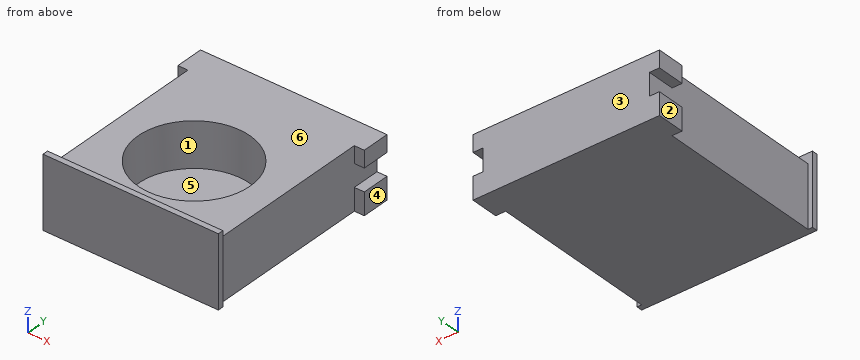
from build123d import *

# Parameters (mm, degrees)
F0_W     = 18.923
F0_H     = 6.985
F1_DEPTH = 22.86
F3_DEPTH = 0.635
F4_R     = 6.35
F5_DEPTH = 5.08
F4_W     = 1.143
F4_H     = 3.175
F6_DEPTH = 6.985
F7_W     = 1.143
F7_H     = 2.54
F8_DEPTH = 12.7


with BuildPart() as f1:
    # F0 (on Front) → F1 (new body)
    with BuildSketch(Plane.XZ):
        with Locations((0, -0.3175)):
            Rectangle(F0_W, F0_H)
    extrude(amount=F1_DEPTH)

    # F2 (on face) → F3 (join)
    with BuildSketch(Plane.XZ.offset(22.86)):
        Polygon((9.976428, 4.318), (-9.9695, 4.318), (-9.9695, -3.81), (-9.4615, -3.81), (-9.4615, 3.175), (9.4615, 3.175), (9.4615, -3.81), (9.976428, -3.81), align=None)
    extrude(amount=-F3_DEPTH)

    # F4 (on face) → F5 (cut)
    with BuildSketch(Plane.XY.offset(3.175)):
        with Locations((0, -13.97)):
            Circle(F4_R)
    extrude(amount=-F5_DEPTH, mode=Mode.SUBTRACT)

    # F4 (on face) → F6 (join, through all)
    with BuildSketch(Plane.XY.offset(3.175)):
        with Locations((-10.033, -1.5875)):
            Rectangle(F4_W, F4_H)
        with Locations((10.033, -1.5875)):
            Rectangle(F4_W, F4_H)
    extrude(amount=-F6_DEPTH)

    # F7 (on face) → F8 (cut)
    with BuildSketch(Plane.XZ):
        with Locations((10.033, 0)):
            Rectangle(F7_W, F7_H)
        with Locations((-10.033, 0)):
            Rectangle(F7_W, F7_H)
    extrude(amount=F8_DEPTH, mode=Mode.SUBTRACT)


solid = f1.part
Verification items for the finished model (mm, model axes). Face numbers are marked on the shaded views. A direction names the side the tool comes from. Give positions to 0.01 mm unless a question says otherwise; leave off trailing zeros. Order: outer loops, then holes, each group sorted by start corner. A loop starts at its lowest first (then second) coordinate and runs counter-clockwise, first axis right, second up. Notation, with made-up numbers: M -39,-3.75 L 11,-3.75 A11 ccw 11,14.25 Z; hole C -12.5,79.25 d8. An arc over 180 degrees is marked long. Answer as a JSON object with one key per item and string values. Group by question number.
1) Cross-section at D-D (x = -8.75). Enter the section's corners in (y, z) (3 decimals).
2) Depth check by flat-ended pin: pin 1 Ø1.3 at (x, z) = (10, -3) entering from -Y; pin 2 Ø4 at (y, z) = (-17.5, -2.5) entering from +X; pin 3 Ø0.6 at (x, y) = (10, -2) entering from +Z (3 decimals); pin 4 Ø1.5 at (y, z) = (-8.5, -3) entering from -X. Enter the tip coordinate at first touch or a pass-through.
3) Cross-section at A-A (x = 0). Enter the section's corners in (y, z) (3 decimals), then the cut area to 3 significant figures.
4) Access from +Z, -Z, +X, -X, +Y, -Y to the whole of each face (thin tool, end or side, straight path). Record for the marked faces 4, 5 and 6.
5) Mould release check, pull along X, two halves, no side actions. Record for the marked faces 1, 2 and 3: released by +X, released by -X, zero draft, split by the parting line, or undercut.
6) Cross-section at B-B (y = -9.5). Enter the section's corners in (x, z) (1 decimal), then the cut area to 3 significant figures.
7) Scan lines: line 1 along X through (y, z) = (-14.25, 0.75); line 2 along Y through (x, z) = (0, 1.75); line 3 along Z through (x, y) = (7, -10) (3 decimals). Record each from-to range of solid material in increasing order. Write a range as [from, to].
Result sheet:
{
 "1": {"outline": "M -22.86,-3.81 L 0,-3.81 L 0,3.175 L -22.225,3.175 L -22.225,4.318 L -22.86,4.318 Z"},
 "2": {"pin 1": "stops at y = -22.86", "pin 2": "stops at x = 9.46", "pin 3": "stops at z = 3.175", "pin 4": "stops at x = -9.46"},
 "3": {"outline": "M -22.86,-3.81 L 0,-3.81 L 0,3.175 L -7.62,3.175 L -7.62,-1.905 L -20.32,-1.905 L -20.32,3.175 L -22.225,3.175 L -22.225,4.318 L -22.86,4.318 Z", "area": "95.9 mm2"},
 "4": {"face 4": "+Z, -Z, +X, +Y, -Y", "face 5": "+Z", "face 6": "+Z, +X, -X, +Y"},
 "5": {"face 1": "undercut", "face 2": "released by -X", "face 3": "zero draft"},
 "6": {"outline": "M -9.5,-3.8 L 9.5,-3.8 L 9.5,3.2 L 4.5,3.2 L 4.5,-1.9 L -4.5,-1.9 L -4.5,3.2 L -9.5,3.2 Z", "area": "86.4 mm2"},
 "7": {"line 1": "x = [-9.46, -6.34], [6.34, 9.46]", "line 2": "y = [-22.86, -20.32], [-7.62, 0]", "line 3": "z = [-3.81, 3.175]"}
}
